Read the model definition and answer for the solid it produces. Units are mm, in the model's axes. Face numbers are marked on the shaded views. A direction names the side the tool comes from. Coordinates: 2 decimals unless noted, no trailing zeros. Write each loop counter-clockwise with the first axis right and the second up, starting at its lowest first coordinate (ties: lowest second). Pieces come first, ordered by that corner, then holes. Notation, with made-up numbers: (51, -20) -> (76, -20) arc R16 cw to (76, 7) -> close; hole circle Ø6 at (-17, 80). An arc over 180 degrees is marked (long way). Return JSON: item names as keys, results as strings.
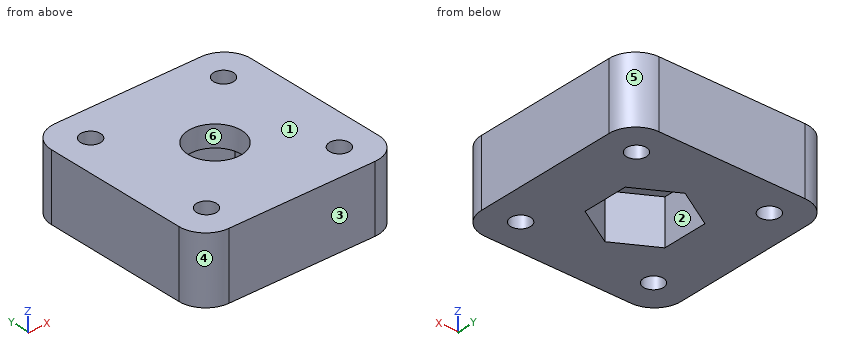
from build123d import *

# Parameters (mm, degrees)
SKETCH_1_W          = 30
SKETCH_1_H          = 30
SKETCH_1_R          = 1.5
SKETCH_1_R_2        = 4
EXTRUDE_1_DEPTH     = 10
CUT_EXTRUDE_1_DEPTH = 6.8
FILLET_1_R          = 4


with BuildPart() as part:
    # Sketch 1 → Extrude 1 (new body)
    with BuildSketch(Plane.XY):
        Rectangle(SKETCH_1_W, SKETCH_1_H)
        with Locations((-10, 10)):
            Circle(SKETCH_1_R, mode=Mode.SUBTRACT)
        with Locations((10, 10)):
            Circle(SKETCH_1_R, mode=Mode.SUBTRACT)
        with Locations((10, -10)):
            Circle(SKETCH_1_R, mode=Mode.SUBTRACT)
        with Locations((-10, -10)):
            Circle(SKETCH_1_R, mode=Mode.SUBTRACT)
        Circle(SKETCH_1_R_2, mode=Mode.SUBTRACT)
    extrude(amount=EXTRUDE_1_DEPTH)

    # Sketch 1_3 → Cut-Extrude 1 (cut)
    with BuildSketch(Plane.XY):
        Polygon((6, 3.464101615), (0, 6.92820323), (-6, 3.464101615), (-6, -3.464101615), (0, -6.92820323), (6, -3.464101615), align=None)
    extrude(amount=CUT_EXTRUDE_1_DEPTH, mode=Mode.SUBTRACT)

    # Fillet 1
    fillet_1_edges = [part.edges().sort_by_distance(p)[0] for p in [
        (-15, -15, 5),
        (-15, 15, 5),
        (15, 15, 5),
        (15, -15, 5),
    ]]
    fillet(fillet_1_edges, radius=FILLET_1_R)


solid = part.part
1. The part is cut by section D-D (z = 1.5). Determine the outline of the cut face in (x, y).
Taken from the geometry:
{"outline": "(-15, -11) arc R4 ccw to (-11, -15) -> (11, -15) arc R4 ccw to (15, -11) -> (15, 11) arc R4 ccw to (11, 15) -> (-11, 15) arc R4 ccw to (-15, 11) -> close; hole circle Ø3 at (-10, -10); hole circle Ø3 at (-10, 10); hole (-6, -3.46) -> (0, -6.93) -> (6, -3.46) -> (6, 3.46) -> (0, 6.93) -> (-6, 3.46) -> close; hole circle Ø3 at (10, -10); hole circle Ø3 at (10, 10)"}
2. The part is cut by section A-A (y = 10). Determine the outline of the cut face in (x, z), then the cut area to 3 significant figures.
Taken from the geometry:
{"outline": "(-15, 0) -> (-11.5, 0) -> (-11.5, 10) -> (-15, 10) -> close; (-8.5, 0) -> (8.5, 0) -> (8.5, 10) -> (-8.5, 10) -> close; (11.5, 0) -> (15, 0) -> (15, 10) -> (11.5, 10) -> close", "area": "240 mm2"}
3. A flat-ended cylindrical pin translates along its axis: pin 1 Ø9.5 at (x, y) = (0.5, -0.5) entering from -Z. Find the tip coordinate at first contact, or state that the pin passes through.
Taken from the geometry:
{"pin 1": "stops at z = 6.8"}
4. For a pull along X with two mould halves and no side action, classify the marked faces 3, 4, 5 and 6 as +X half, -X half, draft (parallel to the pull), parting line (faces both ways), or undercut.
Taken from the geometry:
{"face 3": "draft", "face 4": "-X half", "face 5": "+X half", "face 6": "undercut"}
5. A tool of negligible diameter and unlimited length cuts with its end or side. For the marked faces 1 and 2, from which of +Z, -Z, +X, -X, +Y, -Y can it reach the whole face along a straight path? Write none if from no direction.
Taken from the geometry:
{"face 1": "+Z, +X, -X, +Y, -Y", "face 2": "-Z"}
6. Consider L1, parallel to Y at x = 10, z = 8.25; L2, parallel to X at y = 2.75, z = 5.25; L3, parallel to X at y = 10.75, z = 4.75. Determine where each line is inside the solid, lowest interval first.
Taken from the geometry:
{"L1": "y = -15 to -11.5, -8.5 to 8.5, 11.5 to 15", "L2": "x = -15 to -6, 6 to 15", "L3": "x = -15 to -11.3, -8.7 to 8.7, 11.3 to 15"}
7. The part is cut by section C-C (y = 2.5). Determine the outline of the cut face in (x, z), then the cut area to 3 significant figures.
Taken from the geometry:
{"outline": "(-15, 0) -> (-6, 0) -> (-6, 6.8) -> (-3.12, 6.8) -> (-3.12, 10) -> (-15, 10) -> close; (3.12, 6.8) -> (6, 6.8) -> (6, 0) -> (15, 0) -> (15, 10) -> (3.12, 10) -> close", "area": "198 mm2"}
